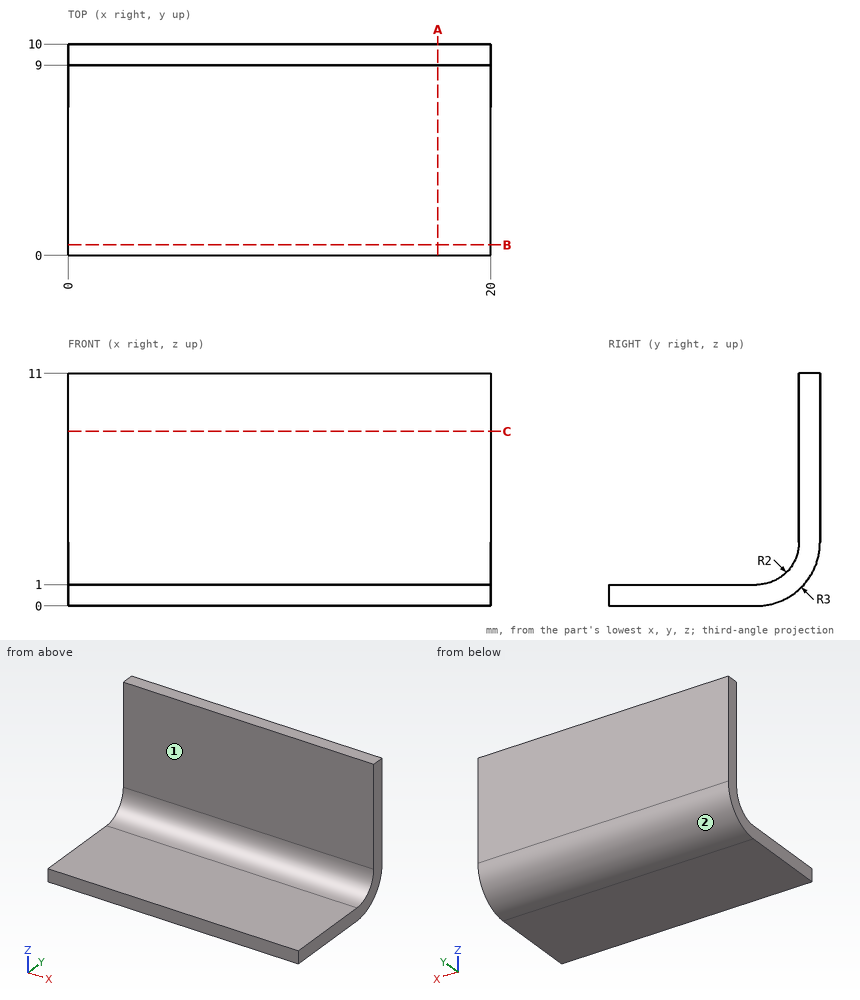
Input: dimensioned drawing with shaded views. Units: mm. Origin: part minimum x, y, z. A direction names the side the tool comes from. Coordinates: 2 decimals unless noted, no trailing zeros. Order: outer loops, then holes, each group sorted by start corner. A loop starts at its lowest first (then second) coordinate and runs counter-clockwise, first axis right, second up. Notation, with made-up numbers: (42.5, 66.25) - (75.5, 66.25) arc R23 cw to (75.5, 77.25) - close; hole circle Ø9 at (7, 0). An arc over 180 degrees is marked (long way). Return JSON: item names as keys, results as strings. Group by question number.
1. Cut plane A-A (x = 17.5). Output: boundary loops of the cut face in (y, z), plus the area to 3 significant figures.
2. Material intervals for line 1 along Y through (x, z) = (2, 3.25); line 2 along Z through (x, y) = (9.25, 0.5); line 3 along Y through (x, z) = (3.25, 2), sorted ascending. Write a range as [from, to].
3. Set-up query: the marked faces 1 and 2. Return all of +Z, -Z, +X, -X, +Y, -Y with unobstructed straight access to the full face (end or side cutting, diameter ignored); none if empty.
4. Cut plane B-B (y = 0.5). Output: boundary loops of the cut face in (x, z).
5. Pin query (flat end, axial travel): pin 1 (5 mm diameter, centred on x = 12, y = 4, fed in from +Z); pin 2 (5.5 mm diameter, centred on x = 9.5, y = 5, fed in from +Z); pin 3 (1 mm diameter, centred on x = 10.5, z = 3, fed in from -Y). Return the tip coordinate at first contact, or that it passes through.
6. Cut plane C-C (z = 8.25). Output: boundary loops of the cut face in (x, y), plus the area to 3 significant figures.
Resolved:
{
 "1": {"outline": "(0, 0) - (7, 0) arc R3 ccw to (10, 3) - (10, 11) - (9, 11) - (9, 3) arc R2 cw to (7, 1) - (0, 1) - close", "area": "18.9 mm²"},
 "2": {"line 1": "y = [9, 10]", "line 2": "z = [0, 1]", "line 3": "y = [8.73, 9.83]"},
 "3": {"face 1": "+Z, +X, -X, -Y", "face 2": "-Z, +X, -X, +Y"},
 "4": {"outline": "(0, 0) - (20, 0) - (20, 1) - (0, 1) - close"},
 "5": {"pin 1": "stops at z = 1", "pin 2": "stops at z = 1.15", "pin 3": "stops at y = 8.94"},
 "6": {"outline": "(0, 9) - (20, 9) - (20, 10) - (0, 10) - close", "area": "20.0 mm²"}
}
